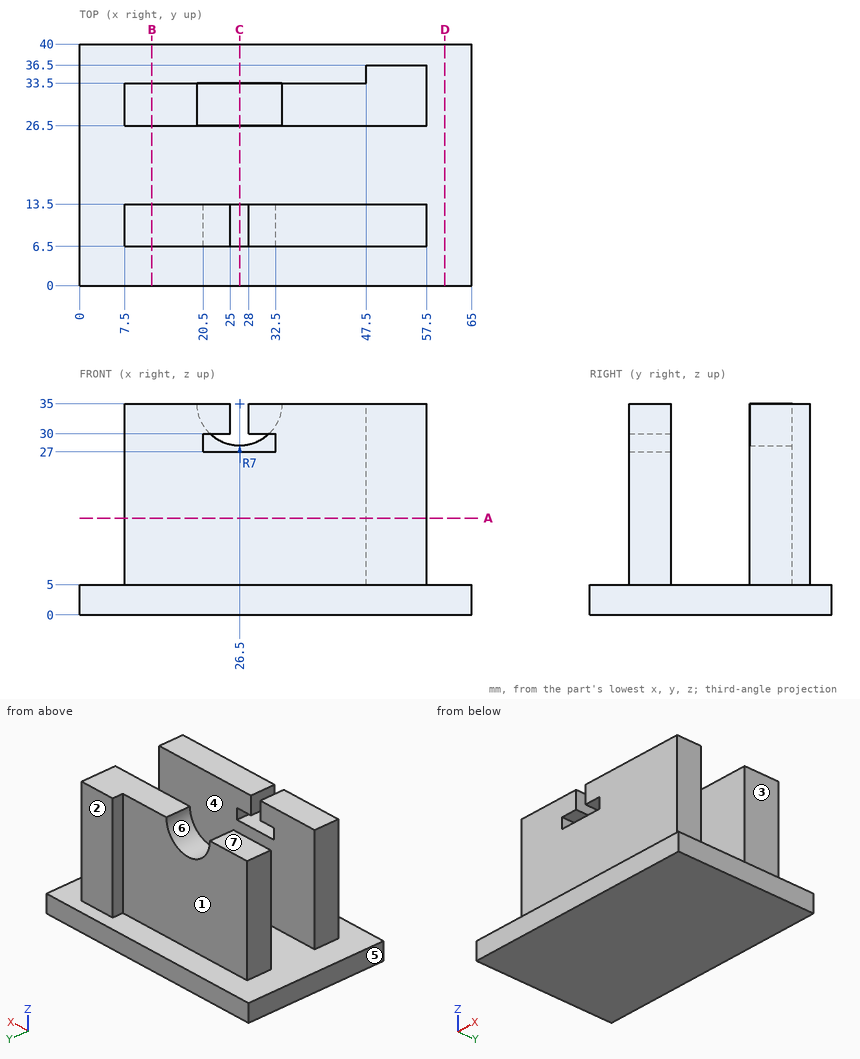
Check sheet for the drawn part. Datum: minimum x, y, z corner. Units: mm. A direction names the side the tool comes from. Give positions to 0.01 mm unless a question says otherwise; leave off trailing zeros. Loops run counter-clockwise (first coordinate to the right, second up) from the corner with the lowest first, then second, coordinate; pieces in that order, holes last. Notation, with made-up numbers: (14, 62) - (42, 62) arc R12 ccw to (42, 80) - close; hole circle Ø2 at (64.5, -14). An arc over 180 degrees is marked (long way). Write each question's results on one line, items separated by ' | '.
1) Depth check by flat-ended pin: P1, Ø3, axis at y = 12.5, z = 14, coming from the -X side; P2, Ø10, axis at x = 10.5, z = 11.5, coming from the -Y side; P3, Ø9, axis at x = 21, z = 19, coming from the +Y side. Enter the tip coordinate at first touch or a pass-through.
Solution:
P1: x = 7.5 | P2: y = 6.5 | P3: y = 33.5
2) Sectioned sample at D-D on x = 60.5. Record the boundary of the cut face in (y, z), plus the area to 3 significant figures.
Solution:
outline: (0, 0) - (40, 0) - (40, 5) - (0, 5) - close | area: 200 mm2
3) Material ranges on L1, parallel to Y at x = 54, z = 14; L2, parallel to Y at x = 32, z = 20.5; L3, parallel to Z at x = 11, y = 15, recorded low to high. Write a range as from..to.
Solution:
L1: 6.5..13.5, 26.5..36.5 | L2: 6.5..13.5, 26.5..33.5 | L3: 0..5
4) Sectioned sample at A-A on z = 16. Record the boundary of the cut face in (x, y).
Solution:
outline: (7.5, 6.5) - (57.5, 6.5) - (57.5, 13.5) - (7.5, 13.5) - close; (7.5, 26.5) - (57.5, 26.5) - (57.5, 36.5) - (47.5, 36.5) - (47.5, 33.5) - (7.5, 33.5) - close
5) Tool access check on the marked faces 1, 2, 3 and 4. Record the directions out of +Z, -Z, +X, -X, +Y, -Y that give a thin tool (end or side, any length) a straight path to the whole face; none if there is none.
Solution:
face 1: +Z, -X, +Y | face 2: +Z, +X, -X, +Y | face 3: +Z, +X, +Y, -Y | face 4: +Z, +X, -X
6) Mould release check, pull along X, two halves, no side actions. Record for the marked faces 5, 6 and 7: pulls with the +X half, pulls with the -X half, needs draft (parallel to the pull), parting line crosses it, or undercut.
Solution:
face 5: pulls with the -X half | face 6: undercut | face 7: needs draft
7) Sectioned sample at C-C on x = 26.5. Record the boundary of the cut face in (y, z).
Solution:
outline: (0, 0) - (40, 0) - (40, 5) - (33.5, 5) - (33.5, 28) - (26.5, 28) - (26.5, 5) - (13.5, 5) - (13.5, 27) - (6.5, 27) - (6.5, 5) - (0, 5) - close
8) Sectioned sample at B-B on x = 12. Record the boundary of the cut face in (y, z), plus the area to 3 significant figures.
Solution:
outline: (0, 0) - (40, 0) - (40, 5) - (33.5, 5) - (33.5, 35) - (26.5, 35) - (26.5, 5) - (13.5, 5) - (13.5, 35) - (6.5, 35) - (6.5, 5) - (0, 5) - close | area: 620 mm2
